Check sheet for the modelled part. Datum: model origin and axes. Units: mm. A direction names the side the tool comes from. Coordinates: 2 decimals unless noted, no trailing zeros. Write each loop counter-clockwise with the first axis right and the second up, starting at its lowest first coordinate (ties: lowest second). Pieces come first, ordered by that corner, then holes. Notation, with made-up numbers: M -6,24 L 27,24 A4 ccw 27,29 Z; hole C 49.25,-35.75 d9. An arc over 180 degrees is marked long. Answer as CSV lines item,"result". Start each with the question number.
Q1. Sectioned sample at C-C, the plane y = -40. Record the cut outline in (x, z), then the cut area to 3 significant figures.
Q2. Access from +Z, -Z, +X, -X, +Y, -Y to the whole of each face (thin tool, end or side, straight path). Record for faces 1 (the flat face through (0, -185, 0)), 2 (the cylindrical face through (-2.05, -47.325, 15.616)).
Q3. Depth check by flat-ended pin: pin 1 Ø6 at (x, z) = (10, 7.5) entering from -Y (3 decimals); pin 2 Ø3 at (x, z) = (10.5, -1) entering from -Y; pin 3 Ø5 at (x, y) = (-8, -118) entering from -Z. Enter the tip coordinate at first touch or a pass-through.
Q4. Sectioned sample at D-D, the plane y = -168.5. Record the cut outline in (x, z) (3 decimals).
Q5. Sectioned sample at A-A, the plane x = 0. Record the cut outline in (y, z) (3 decimals).
Q6. Sectioned sample at B-B, the plane z = 0. Record the cut outline in (x, y) (3 decimals), then the cut area to 3 significant figures.
Q7. Thickness scan on line 1 along Y through (x, z) = (-10, 5.5); line 2 along Z through (x, y) = (-0.5, -101.5); line 3 along Y through (x, z) = (16, 2). Record the ranges inside material, lowest first. Write a range as from..to.
from build123d import *

# Parameters (mm, degrees)
F0_R      = 20
F1_DEPTH  = 35
F3_R      = 15.75
F4_DEPTH  = 25
F6_R      = 13.75
F7_DEPTH  = 50
F8_R      = 12.975
F9_DEPTH  = 25
F10_R     = 11.975
F11_DEPTH = 25
F12_R     = 10.905
F13_DEPTH = 25
F14_SIZE  = 2


with BuildPart() as f1:
    # F0 (on Front) → F1 (new body)
    with BuildSketch(Plane.XZ):
        Circle(F0_R)
    extrude(amount=F1_DEPTH)

    # F3 (on offset) → F4 (join)
    with BuildSketch(Plane.XZ.offset(35)):
        Circle(F3_R)
    extrude(amount=F4_DEPTH)

    # F6 (on offset) → F7 (join)
    with BuildSketch(Plane.XZ.offset(60)):
        Circle(F6_R)
    extrude(amount=F7_DEPTH)

    # F8 (on face) → F9 (join)
    with BuildSketch(Plane.XZ.offset(110)):
        Circle(F8_R)
    extrude(amount=F9_DEPTH)

    # F10 (on face) → F11 (join)
    with BuildSketch(Plane.XZ.offset(135)):
        Circle(F10_R)
    extrude(amount=F11_DEPTH)

    # F12 (on face) → F13 (join)
    with BuildSketch(Plane.XZ.offset(160)):
        Circle(F12_R)
    extrude(amount=F13_DEPTH)

    # F14
    f14_edges = [f1.edges().sort_by_distance(p)[0] for p in [
        (-10.905, -185, 0),
    ]]
    chamfer(f14_edges, length=F14_SIZE)


solid = f1.part
Output:
1,outline,"C 0,0 d31.5"
1,area,"779 mm^2"
2,face 1,"+Z, -Z, +X, -X, -Y"
2,face 2,"-Y"
3,pin 1,"stops at y = -184.405"
3,pin 2,"stops at y = -184.86"
3,pin 3,"stops at z = -11.75"
4,outline,"C 0,0 d21.81"
5,outline,"M -185,-8.905 L -183,-10.905 L -160,-10.905 L -160,-11.975 L -135,-11.975 L -135,-12.975 L -110,-12.975 L -110,-13.75 L -60,-13.75 L -60,-15.75 L -35,-15.75 L -35,-20 L 0,-20 L 0,20 L -35,20 L -35,15.75 L -60,15.75 L -60,13.75 L -110,13.75 L -110,12.975 L -135,12.975 L -135,11.975 L -160,11.975 L -160,10.905 L -183,10.905 L -185,8.905 Z"
6,outline,"M -20,-35 L -15.75,-35 L -15.75,-60 L -13.75,-60 L -13.75,-110 L -12.975,-110 L -12.975,-135 L -11.975,-135 L -11.975,-160 L -10.905,-160 L -10.905,-183 L -8.905,-185 L 8.905,-185 L 10.905,-183 L 10.905,-160 L 11.975,-160 L 11.975,-135 L 12.975,-135 L 12.975,-110 L 13.75,-110 L 13.75,-60 L 15.75,-60 L 15.75,-35 L 20,-35 L 20,0 L -20,0 Z"
6,area,"5,350 mm^2"
7,line 1,"y = -160..0"
7,line 2,"z = -13.74..13.74"
7,line 3,"y = -35..0"
